from build123d import *

# Parameters (mm, degrees)
SKETCH1_W           = 51
SKETCH1_H           = 25.68
BOSS_EXTRUDE1_DEPTH = 20
SKETCH2_W           = 45
SKETCH2_H           = 19.68
CUT_EXTRUDE1_DEPTH  = 17.5
CUT_EXTRUDE5_DEPTH  = 3
SKETCH10_R          = 1.905435321
SKETCH10_W          = 10
SKETCH10_H          = 6
CUT_EXTRUDE6_DEPTH  = 3
SKETCH11_W          = 6.5
SKETCH11_H          = 6.5
SKETCH11_R          = 1.5
BOSS_EXTRUDE4_DEPTH = 18
BOSS_EXTRUDE5_DEPTH = 30


with BuildPart() as part:
    # Sketch1 → Boss-Extrude1 (new body)
    with BuildSketch(Plane(origin=(0, 0, 0), x_dir=(1, 0, 0), z_dir=(0, 1, 0))):
        Rectangle(SKETCH1_W, SKETCH1_H)
    extrude(amount=BOSS_EXTRUDE1_DEPTH)

    # Sketch2 → Cut-Extrude1 (cut)
    with BuildSketch(Plane(origin=(0, 20, 0), x_dir=(1, 0, 0), z_dir=(0, 1, 0))):
        Rectangle(SKETCH2_W, SKETCH2_H)
    extrude(amount=-CUT_EXTRUDE1_DEPTH, mode=Mode.SUBTRACT)

    # Sketch9 → Cut-Extrude5 (cut)
    with BuildSketch(Plane.XY.offset(12.84)):
        with BuildLine():
            Line((-17.5, 20), (17.5, 20))
            ThreePointArc((17.5, 20), (0, 2.5), (-17.5, 20))
        make_face()
    extrude(amount=-CUT_EXTRUDE5_DEPTH, mode=Mode.SUBTRACT)

    # Sketch10 → Cut-Extrude6 (cut)
    with BuildSketch(Plane(origin=(0, 0, -12.84), x_dir=(-1, 0, 0), z_dir=(0, 0, -1))):
        with Locations((0.05, 15.45)):
            Circle(SKETCH10_R)
        with Locations((-17, 17)):
            Rectangle(SKETCH10_W, SKETCH10_H)
    extrude(amount=-CUT_EXTRUDE6_DEPTH, mode=Mode.SUBTRACT)

    # Sketch11 → Boss-Extrude4 (add)
    with BuildSketch(Plane.XZ):
        with Locations((-28.75, 0)):
            Rectangle(SKETCH11_W, SKETCH11_H)
        with Locations((-28.5, 0)):
            Circle(SKETCH11_R, mode=Mode.SUBTRACT)
        with Locations((28.75, 0)):
            Rectangle(SKETCH11_W, SKETCH11_H)
        with Locations((28.5, 0)):
            Circle(SKETCH11_R, mode=Mode.SUBTRACT)
    extrude(amount=-BOSS_EXTRUDE4_DEPTH)

    # Sketch12 → Boss-Extrude5 (add)
    with BuildSketch(Plane.XZ):
        Polygon((-25.5, -3.25), (-25.5, -5.25), (-34, -5.25), (-34, 5.25), (-25.5, 5.25), (-25.5, 3.25), (-32, 3.25), (-32, -3.25), align=None)
        Polygon((25.5, 3.25), (32, 3.25), (32, -3.25), (25.5, -3.25), (25.5, -5.25), (34, -5.25), (34, 5.25), (25.5, 5.25), align=None)
    extrude(amount=-BOSS_EXTRUDE5_DEPTH)


solid = part.part
CAD build for the part. Positions are in the model's coordinates, mm. A direction names the side the tool comes from. Give positions to 0.01 mm unless a question says otherwise; leave off trailing zeros. Write each loop counter-clockwise with the first axis right and the second up, starting at its lowest first coordinate (ties: lowest second). Pieces come first, ordered by that corner, then holes. Notation, with made-up numbers: (52.25, 60.25) - (103.25, 60.25) arc R8 cw to (103.25, 75.25) - close; hole circle Ø6 at (69, 41.5). An arc over 180 degrees is marked (long way). Put each result on its own line as item: value.
(1) Pull direction Z, two halves, no side cores. Call faces 4 (the flat face through (30, 15, -5.25)), 5 (the flat face through (-29, 24, 3.25)), 6 (the cylindrical face through (0.4, 13.6, -11.4)), 7 (the flat face through (-16, 9, 9.84)): released by +Z, released by -Z, zero draft, split by the parting line, or undercut.
Working result:
face 4: released by -Z
face 5: undercut
face 6: zero draft
face 7: undercut
(2) Saw through at A-A (z = 0). List the corners of the cut face in (x, y).
Working result:
outline: (-34, 0) - (-30, 0) - (-30, 18) - (-32, 18) - (-32, 30) - (-34, 30) - close; (-27, 0) - (27, 0) - (27, 18) - (25.5, 18) - (25.5, 20) - (22.5, 20) - (22.5, 2.5) - (-22.5, 2.5) - (-22.5, 20) - (-25.5, 20) - (-25.5, 18) - (-27, 18) - close; (30, 0) - (34, 0) - (34, 30) - (32, 30) - (32, 18) - (30, 18) - close
(3) Saw through at D-D (x = 21). List the corners of the cut face in (y, z).
Working result:
outline: (0, -12.84) - (14, -12.84) - (14, -9.84) - (2.5, -9.84) - (2.5, 9.84) - (20, 9.84) - (20, 12.84) - (0, 12.84) - close
(4) Wall check: L1, parallel to Z at x = -28.5, y = 10.25; L2, parallel to Z at x = 30.5, y = 28.75; L3, parallel to Y at x = -0.05, z = -11.8. Give the ranges that are in metal, low to high.
Working result:
L1: -5.25 to -1.5, 1.5 to 5.25
L2: -5.25 to -3.25, 3.25 to 5.25
L3: 0 to 13.54, 17.36 to 20
(5) Saw through at C-C (x = -28.5). List the corners of the cut face in (y, z), then the cut area to 3 significant figures.
Working result:
outline: (0, -5.25) - (30, -5.25) - (30, -3.25) - (18, -3.25) - (18, -1.5) - (0, -1.5) - close; (0, 1.5) - (18, 1.5) - (18, 3.25) - (30, 3.25) - (30, 5.25) - (0, 5.25) - close
area: 183 mm^2
(6) Saw through at B-B (y = 27.25). List the corners of the cut face in (x, z).
Working result:
outline: (-34, -5.25) - (-25.5, -5.25) - (-25.5, -3.25) - (-32, -3.25) - (-32, 3.25) - (-25.5, 3.25) - (-25.5, 5.25) - (-34, 5.25) - close; (25.5, -5.25) - (34, -5.25) - (34, 5.25) - (25.5, 5.25) - (25.5, 3.25) - (32, 3.25) - (32, -3.25) - (25.5, -3.25) - close
(7) Tool access for faces 1 (the flat face through (12, 17, -11)), 2 (the flat face through (0, 11, -9.84)), 3 (the flat face through (25.5, 10, -9)): list every direction of +Z, -Z, +X, -X, +Y, -Y with a clear straight run to the whole face (end or side of a thin tool).
Working result:
face 1: +Z, -Z, +Y
face 2: +Y
face 3: -Z, +X, +Y, -Y
(8) Drop flat-ended pins along their axis: pin 1 Ø0.9 at (x, z) = (18, -12) entering from +Y; pin 2 Ø8 at (y, z) = (13, 10) entering from +X; pin 3 Ø3.5 at (x, z) = (28.5, 0) entering from +Y. Give the stop position or say it passes through.
Working result:
pin 1: y = 14
pin 2: x = 25.5
pin 3: y = 18
